Geometry: final body of the model. Coordinates: model frame, mm. Face numbers are marked on the shaded views. Coordinates: 2 decimals unless noted, no trailing zeros. Order: outer loops, then holes, each group sorted by start corner. A loop starts at its lowest first (then second) coordinate and runs counter-clockwise, first axis right, second up. Notation, with made-up numbers: M 42,65.25 L 50,65.25 A26 ccw 50,99.25 Z; hole C 20,50 d10. An arc over 180 degrees is marked long. Use CSV: the item, a comma, the result in double quotes. Start each with the question number.
Q1. Mould query, pull axis X, two halves, no side actions, for the marked faces 1, 2 and 3. Classes: +X half, -X half, draft (parallel to the pull), parting line (faces both ways), or undercut.
Q2. Section query D-D, the plane x = -15.5. Output: boundary loops of the cut face in (y, z).
Q3. First-contact query: P1, Ø20.5, axis at x = 0, y = 88.9, coming from the -Z side; P2, Ø3, axis at x = 20, y = -77.5, coming from the -Z side; P3, Ø1.5, axis at x = 15.5, z = 15, coming from the +Y side; P4, Ø2, axis at x = -1, z = 17.5, coming from the -Y side. Flat tips, straight axial feed; report the tip coordinate or a pass-through.
Q4. Section query C-C, the plane z = 6.25. Output: boundary loops of the cut face in (x, y).
Q5. Section query A-A, the plane x = 0. Output: boundary loops of the cut face in (y, z).
Q6. Ray query, probe 1 along Y at (x, z) = (0, 10.5); probe 2 along X at (y, z) = (-88.9, 8.25); probe 3 along Y at (x, z) = (-6.5, 13). Return the intervals inside material, ascending.
Q7. Section query B-B, the plane y = -97. Output: boundary loops of the cut face in (x, z), and give its area (3 significant figures).
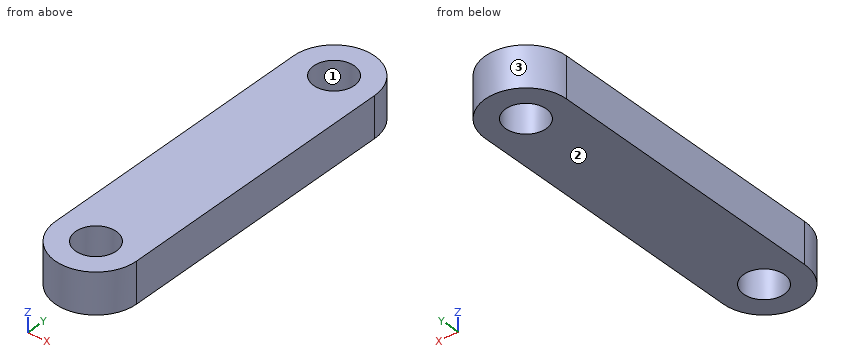
from build123d import *

# Parameters (mm, degrees)
F1_DEPTH = 25.4
F2_R     = 12.7
F3_DEPTH = 25.4


with BuildPart() as f1:
    # F0 (on Top) → F1 (new body)
    with BuildSketch(Plane.XY):
        with BuildLine():
            Line((-25.4, 88.9), (-25.4, 0))
            Line((-25.4, 0), (25.4, 0))
            Line((25.4, 0), (25.4, 88.9))
            ThreePointArc((25.4, 88.9), (0, 63.5), (-25.4, 88.9))
        make_face()
        with BuildLine():
            ThreePointArc((25.4, 88.9), (0, 114.3), (-25.4, 88.9))
            Line((-25.4, 88.9), (25.4, 88.9))
        make_face()
        with BuildLine():
            Line((25.4, 88.9), (-25.4, 88.9))
            ThreePointArc((-25.4, 88.9), (0, 63.5), (25.4, 88.9))
        make_face()
    extrude(amount=F1_DEPTH)

    # F2 (on face) → F3 (cut)
    with BuildSketch(Plane.XY.offset(25.4)):
        with Locations((0, 88.9)):
            Circle(F2_R)
    extrude(amount=-F3_DEPTH, mode=Mode.SUBTRACT)

    # F4: F1 across face


with BuildPart() as f1_1:
    add(f1.part)
    add(f1.part.mirror(Plane(origin=(0, 0, 12.7), x_dir=(1, 0, 0), z_dir=(0, -1, 0))))


solid = f1_1.part
Responses:
1,face 1,"undercut"
1,face 2,"draft"
1,face 3,"parting line"
2,outline,"M -109.02,0 L 109.02,0 L 109.02,25.4 L -109.02,25.4 Z"
3,P1,"passes through"
3,P2,"stops at z = 0"
3,P3,"stops at y = 109.58"
3,P4,"stops at y = -114.3"
4,outline,"M -25.4,-88.9 A25.4 ccw 25.4,-88.9 L 25.4,88.9 A25.4 ccw -25.4,88.9 Z; hole C 0,-88.9 d25.4; hole C 0,88.9 d25.4"
5,outline,"M -114.3,0 L -101.6,0 L -101.6,25.4 L -114.3,25.4 Z; M -76.2,0 L 76.2,0 L 76.2,25.4 L -76.2,25.4 Z; M 101.6,0 L 114.3,0 L 114.3,25.4 L 101.6,25.4 Z"
6,probe 1,"y = -114.3 to -101.6, -76.2 to 76.2, 101.6 to 114.3"
6,probe 2,"x = -25.4 to -12.7, 12.7 to 25.4"
6,probe 3,"y = -113.45 to -99.81, -77.99 to 77.99, 99.81 to 113.45"
7,outline,"M -24.07,0 L -9.78,0 L -9.78,25.4 L -24.07,25.4 Z; M 9.78,0 L 24.07,0 L 24.07,25.4 L 9.78,25.4 Z"
7,area,"726 mm²"
